Check sheet for the modelled part. Datum: model origin and axes. Units: mm. Round coordinates to 2 decimals unless told otherwise and drop trailing zeros. Order: outer loops, then holes, each group sorted by start corner. A loop starts at its lowest first (then second) coordinate and runs counter-clockwise, first axis right, second up. Notation, with made-up numbers: (-8.75, 18.5) -> (17.25, 18.5) arc R35 cw to (17.25, 53.5) -> close; hole circle Ø3 at (17.5, 63.5). An arc over 180 degrees is marked (long way). Answer as CSV lines item,"result". Start each with the question number.
from build123d import *

# Parameters (mm, degrees)
F1_DEPTH = 4
F2_R     = 2.75
F3_DEPTH = 5


with BuildPart() as f1:
    # F0 (on Top) → F1 (new body)
    with BuildSketch(Plane.XY):
        Polygon((175.437126, 97.116617), (-124.562874, 97.116617), (-124.562874, 47.116617), (25.437126, 47.116617), (25.437126, -32.883383), (-124.562874, -32.883383), (-124.562874, -82.883383), (175.437126, -82.883383), (175.437126, -22.883383), (235.437126, -22.883383), (235.437126, 37.116617), (175.437126, 37.116617), align=None)
    extrude(amount=F1_DEPTH)

    # F2 (on face) → F3 (cut)
    with BuildSketch(Plane.XY.offset(4)):
        with Locations((-119.562874, 84.116617)):
            Circle(F2_R)
        with Locations((-65.562874, 84.116617)):
            Circle(F2_R)
        with Locations((-65.562874, 60.116617)):
            Circle(F2_R)
        with Locations((-119.562874, 60.116617)):
            Circle(F2_R)
        with Locations((-119.562874, -45.883383)):
            Circle(F2_R)
        with Locations((-119.562874, -69.883383)):
            Circle(F2_R)
        with Locations((-65.562874, -45.883383)):
            Circle(F2_R)
        with Locations((-65.562874, -69.883383)):
            Circle(F2_R)
    extrude(amount=-F3_DEPTH, mode=Mode.SUBTRACT)


solid = f1.part
1) Section check B-B on z = 0.9. Count the separate pieces of the cut face and the enclosed holes in it, then the cut area to 3 significant figures.
2) Section check D-D on y = 25.5. Record the cut outline in (x, z).
3) Depth check by flat-ended pin: pin 1 Ø7 at (x, y) = (-119.56, 60.12) entering from -Z. Enter the tip coordinate at first touch or a pass-through.
4) Section check A-A on x = 16.5. Record the cut outline in (y, z).
5) Material ranges on line 1 along Y through (x, z) = (-39.5, 1.1); line 2 along X through (y, z) = (69, 2.1); line 3 along X through (y, z) = (-31.5, 3.85), recorded low to high.
6) Section check C-C on x = 181. Record the cut outline in (y, z).
Solutions:
1,separate pieces,"1"
1,enclosed holes,"8"
1,area,"45,400 mm^2"
2,outline,"(25.44, 0) -> (235.44, 0) -> (235.44, 4) -> (25.44, 4) -> close"
3,pin 1,"stops at z = 0"
4,outline,"(-82.88, 0) -> (-32.88, 0) -> (-32.88, 4) -> (-82.88, 4) -> close; (47.12, 0) -> (97.12, 0) -> (97.12, 4) -> (47.12, 4) -> close"
5,line 1,"y = -82.88 to -32.88, 47.12 to 97.12"
5,line 2,"x = -124.56 to 175.44"
5,line 3,"x = 25.44 to 175.44"
6,outline,"(-22.88, 0) -> (37.12, 0) -> (37.12, 4) -> (-22.88, 4) -> close"
